Design review of the part built by this model. Coordinates are the model's own, in mm. A direction names the side the tool comes from. Coordinates: 2 decimals unless noted, no trailing zeros. Order: outer loops, then holes, each group sorted by start corner. A loop starts at its lowest first (then second) coordinate and runs counter-clockwise, first axis right, second up.
from build123d import *

# Parameters (mm, degrees)
BOSS_EXTRUDE1_DEPTH = 2
BOSS_EXTRUDE3_DEPTH = 7
SKETCH1_6_R         = 1.7
BOSS_EXTRUDE4_DEPTH = 7


with BuildPart() as part:
    # Sketch1 → Boss-Extrude1 (new body)
    with BuildSketch(Plane(origin=(0, 0, 0), x_dir=(1, 0, 0), z_dir=(0, 1, 0))):
        Polygon((-4.021978022, 8.267996412), (-4.021978022, 18.267996412), (-16.021978022, 18.267996412), (-16.021978022, -22.732003588), (-4.021978022, -22.732003588), (-2.021978022, -22.732003588), (-2.021978022, -32.732003588), (9.978021978, -32.732003588), (9.978021978, 8.267996412), (-2.021978022, 8.267996412), align=None)
        Polygon((-6.021978022, 6.267996412), (-6.021978022, 16.267996412), (-14.021978022, 16.267996412), (-14.021978022, -20.732003588), (-4.021978022, -20.732003588), (-0.021978022, -20.732003588), (-0.021978022, -30.732003588), (7.978021978, -30.732003588), (7.978021978, 6.267996412), (-2.021978022, 6.267996412), align=None, mode=Mode.SUBTRACT)
    extrude(amount=BOSS_EXTRUDE1_DEPTH)

    # Sketch1_5 → Boss-Extrude3 (add)
    with BuildSketch(Plane(origin=(0, 0, 0), x_dir=(1, 0, 0), z_dir=(0, 1, 0))):
        Polygon((-4.021978022, -24.732003588), (-4.021978022, -34.732003588), (11.978021978, -34.732003588), (11.978021978, 10.267996412), (-2.021978022, 10.267996412), (-2.021978022, 20.267996412), (-18.021978022, 20.267996412), (-18.021978022, -24.732003588), align=None)
        Polygon((-4.021978022, 18.267996412), (-16.021978022, 18.267996412), (-16.021978022, -22.732003588), (-4.021978022, -22.732003588), (-2.021978022, -22.732003588), (-2.021978022, -32.732003588), (9.978021978, -32.732003588), (9.978021978, 8.267996412), (-2.021978022, 8.267996412), (-4.021978022, 8.267996412), align=None, mode=Mode.SUBTRACT)
    extrude(amount=BOSS_EXTRUDE3_DEPTH)

    # Sketch1_6 → Boss-Extrude4 (add)
    with BuildSketch(Plane(origin=(0, 0, 0), x_dir=(1, 0, 0), z_dir=(0, 1, 0))):
        Polygon((-18.021978022, -42.732003588), (11.978021978, -42.732003588), (11.978021978, -34.732003588), (-4.021978022, -34.732003588), (-4.021978022, -24.732003588), (-18.021978022, -24.732003588), align=None)
        with Locations((-3.021978022, -38.732003588)):
            Circle(SKETCH1_6_R, mode=Mode.SUBTRACT)
        Polygon((11.978021978, 28.267996412), (11.978021978, 10.267996412), (-2.021978022, 10.267996412), (-2.021978022, 20.267996412), (-18.021978022, 20.267996412), (-18.021978022, 28.267996412), align=None)
        with Locations((-3.021978022, 24.267996412)):
            Circle(SKETCH1_6_R, mode=Mode.SUBTRACT)
    extrude(amount=BOSS_EXTRUDE4_DEPTH)


solid = part.part
1. Mouldability with a two-part tool opening along Z and no side actions: class faces 1 (the flat face through (-3, 3, -28.268)), 2 (the flat face through (-17, 0, 7)), 3 (the flat face through (-0.022, 1, 26)) as pulls with the +Z half, pulls with the -Z half, needs draft (parallel to the pull), parting line crosses it, or undercut.
2. Add section B-B (z = 17.5). Give the boundary of the cut face in (x, y), and give its area (3 significant figures).
3. Add section D-D (x = 8.75). Give the boundary of the cut face in (y, z), and give its area (3 significant figures).
4. Insertion check: pin 1 (2 mm diameter, centred on x = 8, z = 27, fed in from +Y). The pin has a flat end and moves straight along its axis. Give the tip position at first contact, or say it passes through.
5. Add section A-A (x = -7.75). Give the boundary of the cut face in (y, z).
6. For faces 4 (the flat face through (7.978, 1, 12)), 5 (the flat face through (-9, 4, 22.732)), 6 (the flat face through (-3, 3, 42.732)), list the 3-axis set-ups (+Z, -Z, +X, -X, +Y, -Y) from which the entire face can be reached by the end or side of a thin tool; tool diameter is ignored.
7. Add section C-C (y = 1). Give the boundary of the cut face in (x, z).
8. To check wall thickness, follow line 1 (Z direction, x = -5, y = 5); line 2 (Z direction, x = 6.25, y = 4.5); line 3 (X direction, y = 1.25, z = 20). State the ranges of each line that lie inside material, in increasing order.
Solution:
1. face 1: pulls with the -Z half
1. face 2: needs draft
1. face 3: undercut
2. outline: (-18.02, 0) - (-14.02, 0) - (-14.02, 2) - (-16.02, 2) - (-16.02, 7) - (-18.02, 7) - close; (7.98, 0) - (11.98, 0) - (11.98, 7) - (9.98, 7) - (9.98, 2) - (7.98, 2) - close
2. area: 36.0 mm2
3. outline: (0, -28.27) - (7, -28.27) - (7, -8.27) - (2, -8.27) - (2, 32.73) - (7, 32.73) - (7, 42.73) - (0, 42.73) - close
3. area: 292 mm2
4. pin 1: stops at y = 2
5. outline: (0, -28.27) - (7, -28.27) - (7, -18.27) - (2, -18.27) - (2, -16.27) - (0, -16.27) - close; (0, 20.73) - (2, 20.73) - (2, 22.73) - (7, 22.73) - (7, 42.73) - (0, 42.73) - close
6. face 4: +Y, -Y
6. face 5: +Y
6. face 6: +Z, +X, -X, +Y, -Y
7. outline: (-18.02, -28.27) - (11.98, -28.27) - (11.98, 42.73) - (-18.02, 42.73) - close; hole (-14.02, -16.27) - (-6.02, -16.27) - (-6.02, -6.27) - (7.98, -6.27) - (7.98, 30.73) - (-0.02, 30.73) - (-0.02, 20.73) - (-14.02, 20.73) - close; hole circle Ø3.4 at (-3.02, -24.27); hole circle Ø3.4 at (-3.02, 38.73)
8. line 1: z = -28.27 to -18.27, 22.73 to 42.73
8. line 2: z = -28.27 to -8.27, 32.73 to 42.73
8. line 3: x = -18.02 to -14.02, 7.98 to 11.98
